```python
from build123d import *

# Parameters (mm, degrees)
CBORE_FOR_M8_HEX_SOCKET_THIN_HEAD_CAP_SC_D           = 9
CBORE_FOR_M8_HEX_SOCKET_THIN_HEAD_CAP_SC_DEPTH       = 20
CBORE_FOR_M8_HEX_SOCKET_THIN_HEAD_CAP_SC_CBORE_D     = 15
CBORE_FOR_M8_HEX_SOCKET_THIN_HEAD_CAP_SC_CBORE_DEPTH = 5.6
CBORE_FOR_M8_HEX_SOCKET_THIN_HEAD_CAP_SC_TIP         = 2.703872786
CHAMFER1_SIZE                                        = 0.5


with BuildPart() as part:
    # Sketch1 → Revolve1 (revolve)
    with BuildSketch(Plane.XY, mode=Mode.PRIVATE) as revolve1_sk:
        Polygon((22.938748471, 66.816763283), (42.938748471, 66.816763283), (42.938748471, 3.066763283), (37.938748471, 3.066763283), (37.938748471, 11.816763283), (27.938748471, 11.816763283), (27.938748471, 26.816763283), (21.938748471, 26.816763283), (21.938748471, 36.816763283), (-17.061251529, 36.816763283), (-17.061251529, 41.816763283), (22.938748471, 41.816763283), align=None)
    revolve(revolve1_sk.sketch.rotate(Axis((-15.261904536, -33.183236717, 0), (1, 0, 0)), 90), axis=Axis((-15.261904536, -33.183236717, 0), (1, 0, 0)))

    # CBORE for M8 Hex Socket Thin Head Cap Screw1
    with Locations(Plane(origin=(42.938748471, 0, 0), x_dir=(0, 0, -1), z_dir=(1, 0, 0))):
        with Locations((77.942286341, 11.816763283), (0, 56.816763283), (0, -33.183236717), (-77.942286341, 11.816763283), (-77.942286341, -78.183236717), (0, -123.183236717), (77.942286341, -78.183236717)):
            CounterBoreHole(CBORE_FOR_M8_HEX_SOCKET_THIN_HEAD_CAP_SC_D / 2, CBORE_FOR_M8_HEX_SOCKET_THIN_HEAD_CAP_SC_CBORE_D / 2, CBORE_FOR_M8_HEX_SOCKET_THIN_HEAD_CAP_SC_CBORE_DEPTH, depth=CBORE_FOR_M8_HEX_SOCKET_THIN_HEAD_CAP_SC_DEPTH)
            with Locations((0, 0, -(CBORE_FOR_M8_HEX_SOCKET_THIN_HEAD_CAP_SC_DEPTH + CBORE_FOR_M8_HEX_SOCKET_THIN_HEAD_CAP_SC_TIP / 2))):  # 118° drill point
                Cone(0, CBORE_FOR_M8_HEX_SOCKET_THIN_HEAD_CAP_SC_D / 2, CBORE_FOR_M8_HEX_SOCKET_THIN_HEAD_CAP_SC_TIP, mode=Mode.SUBTRACT)

    # Chamfer1
    chamfer1_edges = [part.edges().sort_by_distance(p)[0] for p in [
        (21.938748471, -33.183236717, -60),
        (-17.061251529, -33.183236717, -70),
        (-17.061251529, -33.183236717, -75),
        (22.938748471, -33.183236717, -100),
        (42.938748471, -33.183236717, -100),
        (42.938748471, -33.183236717, -36.25),
        (37.938748471, -33.183236717, -36.25),
        (27.938748471, -33.183236717, -45),
        (42.938748471, 11.816763283, -70.442286341),
        (22.938748471, 11.816763283, -82.442286341),
        (42.938748471, -78.183236717, -70.442286341),
        (22.938748471, -78.183236717, -82.442286341),
        (42.938748471, -123.183236717, 7.5),
        (22.938748471, -123.183236717, -4.5),
        (22.938748471, -78.183236717, 73.442286341),
        (42.938748471, 11.816763283, 85.442286341),
        (22.938748471, 11.816763283, 73.442286341),
        (42.938748471, 56.816763283, 7.5),
        (22.938748471, 56.816763283, -4.5),
    ]]
    chamfer(chamfer1_edges, length=CHAMFER1_SIZE)


solid = part.part
```
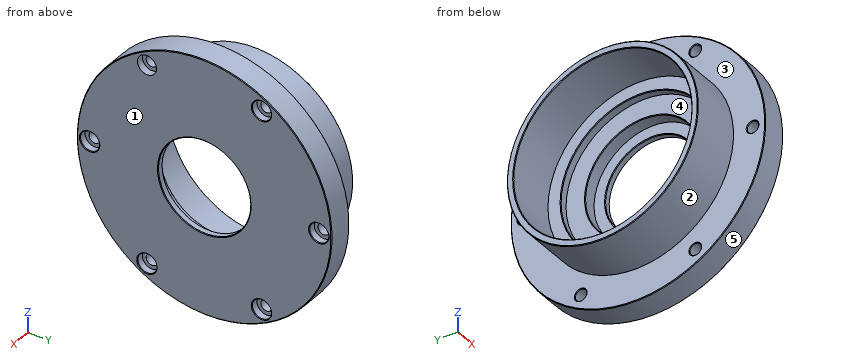
CAD build for the part. Positions are in the model's coordinates, mm. Face numbers are marked on the shaded views. A direction names the side the tool comes from. Give positions to 0.01 mm unless a question says otherwise; leave off trailing zeros. Write each loop counter-clockwise with the first axis right and the second up, starting at its lowest first coordinate (ties: lowest second). Pieces come first, ordered by that corner, then holes. Notation, with made-up numbers: (-29, 44) -> (-21, 44) arc R20 ccw to (-21, 76) -> close; hole circle Ø7 at (85.25, -22). An arc over 180 degrees is marked (long way). Write each question's results on one line, items separated by ' | '.
1. Which spindle directions (+Z, -Z, +X, -X, +Y, -Y) get a long thin tool onto all of the face, cutting with end or side? Do the marked faces 1 and 2. Say none if no direction does.
Geometry check:
face 1: +Z, -Z, +X, +Y, -Y | face 2: -X
2. Cut at B-B, the plane x = 12. Write the cut outline in (y, z).
Geometry check:
outline: circle Ø150 at (-33.18, 0); hole circle Ø140 at (-33.18, 0)
3. Drop flat-ended pins along their axis: P1, Ø10, axis at y = -98.5, z = -70, coming from the -X side; P2, Ø4.5, axis at y = 9.5, z = 81, coming from the +X side; P3, Ø5.5, axis at y = 11.82, z = 77.94, coming from the +X side; P4, Ø12, axis at x = 4.5, z = 65, coming from the -Y side. Give the stop position or say it passes through.
Geometry check:
P1: x = 22.94 | P2: x = 37.34 | P3: through | P4: y = -79.49
4. Wall check: probe 1 along Y at (x, z) = (41.4, 0); probe 2 along Y at (x, z) = (31, 0); probe 3 along Z at (x, y) = (35.5, 8.5). Give the ranges that are in metal, low to high. Write a range as [from, to].
Geometry check:
probe 1: [-133.18, -130.68], [-115.68, -69.43], [3.07, 49.32], [64.32, 66.82] | probe 2: [-133.18, -127.68], [-118.68, -78.18], [11.82, 52.32], [61.32, 66.82] | probe 3: [-90.9, -80.98], [-74.9, -16.96], [16.96, 74.9], [80.98, 90.9]
5. Two-plate mould, pull along Y, no slides. Class the marked faces 3, 4 and 5: pulls with the +Y half, pulls with the -Y half, needs draft (parallel to the pull), parting line crosses it, or undercut.
Geometry check:
face 3: needs draft | face 4: undercut | face 5: parting line crosses it
6. Cut at A-A, the plane z = 0. Give the number of separate pieces and of enclosed holes in the cut face, then the cut area to 3 significant figures.
Geometry check:
separate pieces: 4 | enclosed holes: 0 | area: 2,130 mm²
